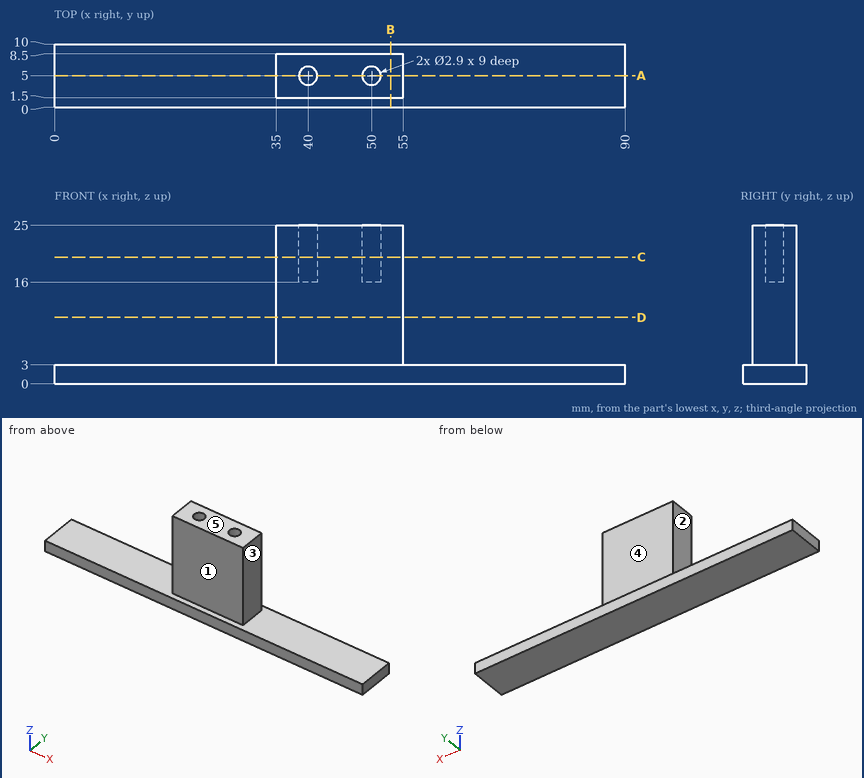
Part print with two shaded views. Sizes in mm from the minimum x, y, z corner. A direction names the side the tool comes from. Give positions to 0.01 mm unless a question says otherwise; leave off trailing zeros. Order: outer loops, then holes, each group sorted by start corner. A loop starts at its lowest first (then second) coordinate and runs counter-clockwise, first axis right, second up.
1) Saw through at C-C, the plane z = 20. Write the cut outline in (x, y), then the cut area to 3 significant figures.
2) 3-axis set-ups, long thin cutter, end or side, ignore diameter. For the marked faces 1, 2, 3, 4 and 5: which of +Z, -Z, +X, -X, +Y, -Y reach the whole face in a straight line?
3) Pin check, flat tips, straight feed: pin 1 (1.5 mm diameter, centred on x = 40, y = 5.5, fed in from +Z); pin 2 (10 mm diameter, centred on x = 40.5, z = 16, fed in from -Y); pin 3 (3 mm diameter, centred on x = 27.5, y = 4.5, fed in from +Z). Stop position of each tip, or through.
4) Saw through at D-D, the plane z = 10.5. Write the cut outline in (x, y), then the cut area to 3 significant figures.
5) Saw through at A-A, the plane y = 5. Write the cut outline in (x, z), then the cut area to 3 significant figures.
6) Saw through at B-B, the plane x = 53. Write the cut outline in (y, z).
7) Wall check: probe 1 along X at (y, z) = (5, 18.75); probe 2 along Y at (x, z) = (40, 19.25); probe 3 along X at (y, z) = (6, 10.75). Give the ranges that are in metal, low to high.
Computed:
1. outline: (35, 1.5) - (55, 1.5) - (55, 8.5) - (35, 8.5) - close; hole circle Ø2.9 at (40, 5); hole circle Ø2.9 at (50, 5)
1. area: 127 mm2
2. face 1: +Z, +X, -X, -Y
2. face 2: +Z, -X, +Y, -Y
2. face 3: +Z, +X, +Y, -Y
2. face 4: +Z, +X, -X, +Y
2. face 5: +Z, +X, -X, +Y, -Y
3. pin 1: stops at z = 16
3. pin 2: stops at y = 1.5
3. pin 3: stops at z = 3
4. outline: (35, 1.5) - (55, 1.5) - (55, 8.5) - (35, 8.5) - close
4. area: 140 mm2
5. outline: (0, 0) - (90, 0) - (90, 3) - (55, 3) - (55, 25) - (51.45, 25) - (51.45, 16) - (48.55, 16) - (48.55, 25) - (41.45, 25) - (41.45, 16) - (38.55, 16) - (38.55, 25) - (35, 25) - (35, 3) - (0, 3) - close
5. area: 658 mm2
6. outline: (0, 0) - (10, 0) - (10, 3) - (8.5, 3) - (8.5, 25) - (1.5, 25) - (1.5, 3) - (0, 3) - close
7. probe 1: x = 35 to 38.55, 41.45 to 48.55, 51.45 to 55
7. probe 2: y = 1.5 to 3.55, 6.45 to 8.5
7. probe 3: x = 35 to 55
